Part model, mm, in its own coordinate system. Face numbers are marked on the shaded views. A direction names the side the tool comes from. Coordinates: 2 decimals unless noted, no trailing zeros. Loops run counter-clockwise (first coordinate to the right, second up) from the corner with the lowest first, then second, coordinate; pieces in that order, holes last. Notation, with made-up numbers: M 3.5,6 L 37.5,6 A21 cw 37.5,31 Z; hole C -22.5,74 d3. An arc over 180 degrees is marked long. Answer as CSV lines item,"result". Start each with the question number.
from build123d import *

# Parameters (mm, degrees)
F1_DEPTH = 38.1
F3_DEPTH = 25.4
F5_DEPTH = 4.2333333333
F7_DEPTH = 4.2333333333
F9_D     = 7.62
F9_DEPTH = 12.7
F9_TIP   = 2.2892789585


with BuildPart() as f1:
    # F0 (on Right) → F1 (new body)
    with BuildSketch(Plane.YZ):
        Polygon((-31.7897086839, 80.859287534), (-36.0230420173, 80.859287534), (-36.0230420173, -46.140712466), (40.1769579827, -46.140712466), (40.1769579827, -41.9073791327), (-31.7897086839, -41.9073791327), align=None)
    extrude(amount=F1_DEPTH)

    # F2 (on face) → F3 (cut)
    with BuildSketch(Plane.XZ.offset(36.0230420173)):
        with BuildLine():
            Line((21.844, 61.4068451581), (16.256, 61.4068451581))
            ThreePointArc((16.256, 61.4068451581), (13.7415282861, 60.365316872), (12.7, 57.8508451581))
            ThreePointArc((12.7, 57.8508451581), (13.7415282861, 55.3363734442), (16.256, 54.2948451581))
            Line((16.256, 54.2948451581), (21.844, 54.2948451581))
            ThreePointArc((21.844, 54.2948451581), (24.3584717139, 55.3363734442), (25.4, 57.8508451581))
            ThreePointArc((25.4, 57.8508451581), (24.3584717139, 60.365316872), (21.844, 61.4068451581))
        make_face()
    extrude(amount=-F3_DEPTH, mode=Mode.SUBTRACT)

    # F4 (on face) → F5 (join)
    with BuildSketch(Plane.YZ.offset(38.1)):
        Polygon((-31.7897086839, -41.9073791327), (-6.3897086839, -41.9073791327), (-31.7897086839, -16.5073791327), align=None)
    extrude(amount=-F5_DEPTH)

    # F6 (on face) → F7 (join)
    with BuildSketch(Plane(origin=(0, 0, 0), x_dir=(0, -1, 0), z_dir=(-1, 0, 0))):
        Polygon((31.7897086839, -41.9073791327), (31.7897086839, -16.5073791327), (6.3897086839, -41.9073791327), align=None)
    extrude(amount=-F7_DEPTH)

    # F9
    with Locations(Plane.XY.offset(-41.9073791327)):
        with Locations((19.05, 0), (19.05, 29.5239835978)):
            Hole(F9_D / 2, depth=F9_DEPTH)
            with Locations((0, 0, -(F9_DEPTH + F9_TIP / 2))):  # 118° drill point
                Cone(0, F9_D / 2, F9_TIP, mode=Mode.SUBTRACT)


solid = f1.part
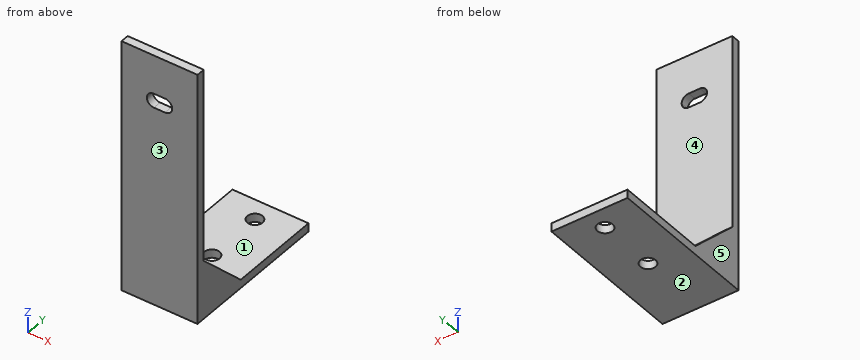
Q1. Slice it at C-C, the plane x = 36.5. Write the cut outline in (y, z).
Q2. Slice it at B-B, the plane y = 0. Write the cut outline in (x, z), and give its area (3 significant figures).
Q3. Wall check: L1, parallel to Y at x = 19, z = -44; L2, parallel to Z at x = 20, y = 22; L3, parallel to Y at x = 18, z = 48. Give the ranges that are in metal, low to high.
Q4. Tool access for the marked faces 1 and 2: list every direction of +Z, -Z, +X, -X, +Y, -Y with a clear straight run to the whole face (end or side of a thin tool).
Q5. Slice it at D-D, the plane z = -23. Write the cut outline in (x, y).
Q6. Flat gauge pins, fed straight in: P1, Ø12, axis at x = 19.05, y = 0, coming from the +Z side; P2, Ø6, axis at x = 19.05, y = 29.52, coming from the +Z side; P3, Ø19, axis at x = 12.5, z = 35.5, coming from the +Y side; P4, Ø7.5, axis at y = -20, z = -30, coming from the -X side. Where does each tip first touch, or does it go through?
Q7. Slice it at A-A, the plane x = 19.05. Write the cut outline in (y, z).
Q8. Two-plate mould, pull along X, no slides. Class the marked faces 3, 4 and 5: +X half, -X half, draft (parallel to the pull), parting line (faces both ways), or undercut.
Solved:
1,outline,"M -36.02,-46.14 L 40.18,-46.14 L 40.18,-41.91 L -6.39,-41.91 L -31.79,-16.51 L -31.79,80.86 L -36.02,80.86 Z"
2,outline,"M 0,-46.14 L 15.24,-46.14 L 15.24,-41.91 L 0,-41.91 Z; M 22.86,-46.14 L 38.1,-46.14 L 38.1,-41.91 L 22.86,-41.91 Z"
2,area,"129 mm2"
3,L1,"y = -36.02 to -3.81, 3.81 to 25.71, 33.33 to 40.18"
3,L2,"z = -46.14 to -41.91"
3,L3,"y = -36.02 to -31.79"
4,face 1,"+Z, +Y"
4,face 2,"-Z, +X, -X, +Y, -Y"
5,outline,"M 0,-36.02 L 38.1,-36.02 L 38.1,-25.3 L 33.87,-25.3 L 33.87,-31.79 L 4.23,-31.79 L 4.23,-25.3 L 0,-25.3 Z"
6,P1,"stops at z = -41.91"
6,P2,"passes through"
6,P3,"stops at y = -31.79"
6,P4,"stops at x = 0"
7,outline,"M -36.02,-46.14 L -3.81,-46.14 L -3.81,-41.91 L -31.79,-41.91 L -31.79,54.29 L -36.02,54.29 Z; M -36.02,61.41 L -31.79,61.41 L -31.79,80.86 L -36.02,80.86 Z; M 3.81,-46.14 L 25.71,-46.14 L 25.71,-41.91 L 3.81,-41.91 Z; M 33.33,-46.14 L 40.18,-46.14 L 40.18,-41.91 L 33.33,-41.91 Z"
8,face 3,"draft"
8,face 4,"undercut"
8,face 5,"-X half"
